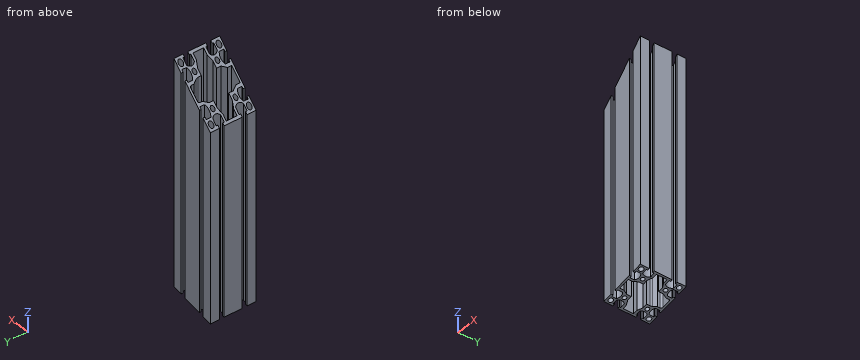
```python
from build123d import *

# Parameters (mm, degrees)
F0_R          = 3
F0_R_2        = 2.5
F1_DEPTH      = 309.2
F2_R          = 2
F3_R          = 7
F6_DEPTH      = 30
F6_DEPTH_BACK = 30


# Not quite as in the source:
# - a feature names something its author has since deleted; it is built from what else it names


with BuildPart() as f1:
    # F0 (on Top) → F1 (new body)
    with BuildSketch(Plane.XY):
        with BuildLine():
            Line((18.15, -30), (30, -30))
            Line((30, -30), (30, -18.15))
            Line((30, -18.15), (27.5, -18.15))
            Line((27.5, -18.15), (27.5, -20.15))
            Line((27.5, -20.15), (21.5477069044, -20.15))
            ThreePointArc((21.5477069044, -20.15), (19.5, -15), (21.5477069044, -9.85))
            Line((21.5477069044, -9.85), (27.5, -9.85))
            Line((27.5, -9.85), (27.5, -11.85))
            Line((27.5, -11.85), (30, -11.85))
            Line((30, -11.85), (30, 11.85))
            Line((30, 11.85), (27.5, 11.85))
            Line((27.5, 11.85), (27.5, 9.85))
            Line((27.5, 9.85), (21.5477069044, 9.85))
            ThreePointArc((21.5477069044, 9.85), (19.5, 15), (21.5477069044, 20.15))
            Line((21.5477069044, 20.15), (27.5, 20.15))
            Line((27.5, 20.15), (27.5, 18.15))
            Line((27.5, 18.15), (30, 18.15))
            Line((30, 18.15), (30, 30))
            Line((30, 30), (18.15, 30))
            Line((18.15, 30), (18.15, 27.5))
            Line((18.15, 27.5), (20.15, 27.5))
            Line((20.15, 27.5), (20.15, 21.5477069044))
            ThreePointArc((20.15, 21.5477069044), (15, 19.5), (9.85, 21.5477069044))
            Line((9.85, 21.5477069044), (9.85, 27.5))
            Line((9.85, 27.5), (11.85, 27.5))
            Line((11.85, 27.5), (11.85, 30))
            Line((11.85, 30), (-11.85, 30))
            Line((-11.85, 30), (-11.85, 27.5))
            Line((-11.85, 27.5), (-9.85, 27.5))
            Line((-9.85, 27.5), (-9.85, 21.5477069044))
            ThreePointArc((-9.85, 21.5477069044), (-15, 19.5), (-20.15, 21.5477069044))
            Line((-20.15, 21.5477069044), (-20.15, 27.5))
            Line((-20.15, 27.5), (-18.15, 27.5))
            Line((-18.15, 27.5), (-18.15, 30))
            Line((-18.15, 30), (-30, 30))
            Line((-30, 30), (-30, 18.15))
            Line((-30, 18.15), (-27.5, 18.15))
            Line((-27.5, 18.15), (-27.5, 20.15))
            Line((-27.5, 20.15), (-21.5477069044, 20.15))
            ThreePointArc((-21.5477069044, 20.15), (-19.5, 15), (-21.5477069044, 9.85))
            Line((-21.5477069044, 9.85), (-27.5, 9.85))
            Line((-27.5, 9.85), (-27.5, 11.85))
            Line((-27.5, 11.85), (-30, 11.85))
            Line((-30, 11.85), (-30, -11.85))
            Line((-30, -11.85), (-27.5, -11.85))
            Line((-27.5, -11.85), (-27.5, -9.85))
            Line((-27.5, -9.85), (-21.5477069044, -9.85))
            ThreePointArc((-21.5477069044, -9.85), (-19.5, -15), (-21.5477069044, -20.15))
            Line((-21.5477069044, -20.15), (-27.5, -20.15))
            Line((-27.5, -20.15), (-27.5, -18.15))
            Line((-27.5, -18.15), (-30, -18.15))
            Line((-30, -18.15), (-30, -30))
            Line((-30, -30), (-18.15, -30))
            Line((-18.15, -30), (-18.15, -27.5))
            Line((-18.15, -27.5), (-20.15, -27.5))
            Line((-20.15, -27.5), (-20.15, -21.5477069044))
            ThreePointArc((-20.15, -21.5477069044), (-15, -19.5), (-9.85, -21.5477069044))
            Line((-9.85, -21.5477069044), (-9.85, -27.5))
            Line((-9.85, -27.5), (-11.85, -27.5))
            Line((-11.85, -27.5), (-11.85, -30))
            Line((-11.85, -30), (11.85, -30))
            Line((11.85, -30), (11.85, -27.5))
            Line((11.85, -27.5), (9.85, -27.5))
            Line((9.85, -27.5), (9.85, -21.5477069044))
            ThreePointArc((9.85, -21.5477069044), (15, -19.5), (20.15, -21.5477069044))
            Line((20.15, -21.5477069044), (20.15, -27.5))
            Line((20.15, -27.5), (18.15, -27.5))
            Line((18.15, -27.5), (18.15, -30))
        make_face()
        with Locations((-25, -25)):
            Circle(F0_R, mode=Mode.SUBTRACT)
        with Locations((-15, -15)):
            Circle(F0_R_2, mode=Mode.SUBTRACT)
        with Locations((25, -25)):
            Circle(F0_R, mode=Mode.SUBTRACT)
        with Locations((15, -15)):
            Circle(F0_R_2, mode=Mode.SUBTRACT)
        with Locations((-25, 25)):
            Circle(F0_R, mode=Mode.SUBTRACT)
        with Locations((-15, 15)):
            Circle(F0_R_2, mode=Mode.SUBTRACT)
        Polygon((-7, 22), (-7, 27.5), (0, 27.5), (7, 27.5), (7, 22), (10, 16), (10, 10), (16, 10), (22, 7), (27.5, 7), (27.5, 0), (27.5, -7), (22, -7), (16, -10), (10, -10), (10, -16), (7, -22), (7, -27.5), (0, -27.5), (-7, -27.5), (-7, -22), (-10, -16), (-10, -10), (-16, -10), (-22, -7), (-27.5, -7), (-27.5, 0), (-27.5, 7), (-22, 7), (-16, 10), (-10, 10), (-10, 16), align=None, mode=Mode.SUBTRACT)
        with Locations((15, 15)):
            Circle(F0_R_2, mode=Mode.SUBTRACT)
        with Locations((25, 25)):
            Circle(F0_R, mode=Mode.SUBTRACT)
    extrude(amount=F1_DEPTH)

    # F2
    f2_edges = [f1.edges().sort_by_distance(p)[0] for p in [
        (-7, 27.5, 154.6),
        (7, 27.5, 154.6),
    ]]
    fillet(f2_edges, radius=F2_R)

    # F3
    f3_edges = [f1.edges().sort_by_distance(p)[0] for p in [
        (-10, 16, 154.6),
        (10, 16, 154.6),
    ]]
    fillet(f3_edges, radius=F3_R)

    # F5 (on Front) → F6 (cut, two sides)
    with BuildSketch(Plane.XZ) as f6_sk:
        Polygon((199.6708250374, -78.6542790774), (175.8796550084, 40.952009573), (-30, 0), (-6.208829971, -119.6062886505), align=None)
        Polygon((30, 309.2), (-52.0743704197, 391.2743704197), (-206.6919281066, 236.6568127329), (-124.6175576868, 154.5824423132), align=None)
    extrude(amount=F6_DEPTH, mode=Mode.SUBTRACT)
    extrude(f6_sk.sketch, amount=-F6_DEPTH_BACK, mode=Mode.SUBTRACT)


solid = f1.part
```
The model under review builds one solid part; all positions refer to its coordinate system, in mm. Give positions to 0.01 mm unless a question says otherwise; leave off trailing zeros. Write each loop counter-clockwise with the first axis right and the second up, starting at its lowest first coordinate (ties: lowest second). Pieces come first, ordered by that corner, then holes. Notation, with made-up numbers: (59.25, 33) - (93.25, 33) arc R15 ccw to (93.25, 38) - close; hole circle Ø4 at (-28, 13). An arc over 180 degrees is marked (long way). Answer in a Markdown table with one row per item. Add a question column.
1. We need section B-B on z = 25. State how many separate pieces and enclosed holes the cut face has, then the cut area to 3 significant figures.
2. Wall thickness on line 1 along X through (y, z) = (-25, 185); line 2 along Y through (x, z) = (14.5, 164.5); line 3 along Y through (x, z) = (15, 85): over which ranges is each line inside the solid? List them lowest first. Write a range as [from, to].
3. Insertion check: P1, Ø5, axis at x = -14, y = -19.5, coming from the +Z side; P2, Ø6.5, axis at x = -15, y = 15, coming from the -Z side; P3, Ø1, axis at y = -17, z = 248.5, coming from the -X side. Each pin has a flat end and moves straight along its axis. Give the tip position at first contact, or say it passes through.
4. We need section A-A on y = 0.5. Write out the cut boundary in (x, z).
Ans:
| question | item | result |
|---|---|---|
| 1 | separate pieces | 1 |
| 1 | enclosed holes | 9 |
| 1 | area | 1,080 mm^2 |
| 2 | line 1 | x = [-30, -28], [-22, -20.15], [-9.85, -7], [7, 9.85], [20.15, 22], [28, 30] |
| 2 | line 2 | y = [-19.52, -17.45], [-12.55, -10], [10, 12.55], [17.45, 19.52] |
| 2 | line 3 | y = [-19.5, -17.5], [-12.5, -10], [10, 12.5], [17.5, 19.5] |
| 3 | P1 | stops at z = 267.7 |
| 3 | P2 | stops at z = 2.34 |
| 3 | P3 | stops at x = -19.93 |
| 4 | outline | (-30, 0) - (-27.5, 0.5) - (-27.5, 251.7) - (-30, 249.2) - close; (27.5, 11.44) - (30, 11.93) - (30, 309.2) - (27.5, 306.7) - close |
